from build123d import *

# Parameters (mm, degrees)
F2_W      = 5.5
F2_H      = 5
F4_W      = 25.4
F4_H      = 25.4
F5_DEPTH  = 50
F6_W      = 10
F6_H      = 5.5
F7_DEPTH  = 25
F8_R      = 4.25
F9_DEPTH  = 50
F10_SIZE  = 1
F12_R     = 6
F13_DEPTH = 25
F15_DEPTH = 40


with BuildPart() as f1:
    # F0 (on Front) → F1 (revolve)
    with BuildSketch(Plane.XZ):
        Polygon((0, 59), (0, 0), (42.5, 0), (42.5, 32), (24, 51.5), (24, 59), align=None)
    revolve(axis=Axis((0, 0, 29.5), (0, 0, -1)))

    # F2 (on Front) → F3 (revolve, cut)
    with BuildSketch(Plane.XZ):
        Polygon((5.5, 35), (0, 35), (0, 25), (8.5, 25), (8.5, 35), align=None)
        with Locations((2.75, 37.5)):
            Rectangle(F2_W, F2_H)
        Polygon((11, 59), (0, 59), (0, 40), (5.5, 40), (11, 40), align=None)
    revolve(axis=Axis((0, 0, 30), (0, 0, -1)), mode=Mode.SUBTRACT)

    # F4 (on Right) → F5 (cut, symmetric)
    with BuildSketch(Plane.YZ):
        with Locations((0, 12.7)):
            Rectangle(F4_W, F4_H)
    extrude(amount=F5_DEPTH, both=True, mode=Mode.SUBTRACT)

    # F6 (on Front) → F7 (cut, symmetric)
    with BuildSketch(Plane.XZ):
        with Locations((0, 56.25)):
            Rectangle(F6_W, F6_H)
    extrude(amount=F7_DEPTH, both=True, mode=Mode.SUBTRACT)

    # F8 (on Front) → F9 (cut)
    with BuildSketch(Plane.XZ):
        with Locations((0, 12.7)):
            Circle(F8_R)
        with Locations((28, 12.7)):
            Circle(F8_R)
        with Locations((-28, 12.7)):
            Circle(F8_R)
    extrude(amount=F9_DEPTH, mode=Mode.SUBTRACT)

    # F10
    f10_edges = [f1.edges().sort_by_distance(p)[0] for p in [
        (0, -42.5, 0),
        (0, 42.5, 0),
        (-24, 0, 59),
        (18.654758, -15.099669, 59),
        (18.654758, 15.099669, 59),
    ]]
    chamfer(f10_edges, length=F10_SIZE)

    # F12 (on offset) → F13 (cut)
    with BuildSketch(Plane.XZ.offset(22.5)):
        with Locations((0, 12.7)):
            Circle(F12_R)
        with Locations((-28, 12.7)):
            Circle(F12_R)
        with Locations((28, 12.7)):
            Circle(F12_R)
    extrude(amount=F13_DEPTH, mode=Mode.SUBTRACT)

    # F14 (on Right) → F15 (cut, symmetric)
    with BuildSketch(Plane.YZ):
        with BuildLine():
            Line((-34, 25), (-49.6562516332, 25))
            Line((-49.6562516332, 25), (-49.6562516332, -7.5937491908))
            Line((-49.6562516332, -7.5937491908), (-28, -7.5937491908))
            Line((-28, -7.5937491908), (-28, 19))
            ThreePointArc((-28, 19), (-29.7573593129, 23.2426406871), (-34, 25))
        make_face()
        with BuildLine():
            Line((49.6562516332, -7.5937491908), (49.6562516332, 25))
            Line((49.6562516332, 25), (34, 25))
            ThreePointArc((34, 25), (29.7573593129, 23.2426406871), (28, 19))
            Line((28, 19), (28, -7.5937491908))
            Line((28, -7.5937491908), (49.6562516332, -7.5937491908))
        make_face()
    extrude(amount=F15_DEPTH, both=True, mode=Mode.SUBTRACT)


solid = f1.part
The listing builds one solid part. Answer for the finished solid, in the listing's coordinates (mm). A direction names the side the tool comes from. Round coordinates to 2 decimals unless told otherwise and drop trailing zeros. Loops run counter-clockwise (first coordinate to the right, second up) from the corner with the lowest first, then second, coordinate; pieces in that order, holes last. Notation, with made-up numbers: M 24.5,84.5 L 83.5,84.5 A32 cw 83.5,114.5 Z; hole C 63.25,-39.75 d11. An arc over 180 degrees is marked long. Write each question's results on one line, items separated by ' | '. Start each with the question number.
1) Each of these flat-tipped pins is pushed along its axis until it touches: pin 1 (3 mm diameter, centred on x = -29.5, z = 15.5, fed in from -Y); pin 2 (5 mm diameter, centred on y = 13, z = 7, fed in from +X); pin 3 (6 mm diameter, centred on y = 16, z = 57.5, fed in from -X); pin 4 (6 mm diameter, centred on x = 16.5, y = 28, fed in from -Z). Where does it stop, or does it pass through?
2) Which of the six approach directions +Z, -Z, +X, -X, +Y, -Y give full straight-line access (tool end or side, diameter ignored) to faces 1 (the flat face through (3, -5, 40)), 2 (the flat face through (0, -17, 53.5)), 3 (the cylindrical face through (24.868, -17.531, 15.572)), 4 (the flat face through (0, 6, 35))?
3) Find section B-B on x = 0. Count the separate pieces of the cut face and the enclosed holes in it, plus the area to 3 significant figures.
4) Find section A-A on y = 0. Write down the section's boundary in (x, z), plus the area to 3 significant figures.
5) Straight lines are drawn through the part: probe 1 along X at (y, z) = (-16.25, 12.7); probe 2 along Y at (x, z) = (-22, 7.5); probe 3 along Z at (x, y) = (-6, -4.5). For each, find the intervals that lie inside material, in ascending order.
6) Determine the mould class of faces 5 (the cylindrical face through (-5.2, 23.43, 54.8)), 6 (the flat face through (0, 37, 25)), 7 (the cylindrical face through (10.492, -3.304, 49.633)) for opening direction Y: pulls with the +Y half, pulls with the -Y half, needs draft (parallel to the pull), parting line crosses it, or undercut.
Final values:
1) pin 1: y = -22.5 | pin 2: x = 40.56 | pin 3: x = -20.17 | pin 4: z = 0
2) face 1: +Z | face 2: +Z, +Y, -Y | face 3: -Y | face 4: -Z
3) separate pieces: 3 | enclosed holes: 0 | area: 2,090 mm²
4) outline: M -42.5,25.4 L -8.5,25.4 L -8.5,35 L -5.5,35 L -5.5,40 L -11,40 L -11,59 L -23,59 L -24,58 L -24,51.5 L -42.5,32 Z; M 5.5,35 L 8.5,35 L 8.5,25.4 L 42.5,25.4 L 42.5,32 L 24,51.5 L 24,58 L 23,59 L 11,59 L 11,40 L 5.5,40 Z | area: 1,580 mm²
5) probe 1: -39.27 to -32.25, -23.75 to -4.25, 4.25 to 23.75, 32.25 to 39.27 | probe 2: -28 to -12.7, 12.7 to 28 | probe 3: 35 to 40
6) face 5: parting line crosses it | face 6: needs draft | face 7: undercut
